Read the model definition and answer for the solid it produces. Units are mm, in the model's axes. A direction names the side the tool comes from. Round coordinates to 2 decimals unless told otherwise and drop trailing zeros. Write each loop counter-clockwise with the first axis right and the second up, starting at its lowest first coordinate (ties: lowest second). Pieces come first, ordered by that corner, then holes. Notation, with made-up numbers: (44.5, 16) -> (99.5, 16) arc R35 cw to (99.5, 55) -> close; hole circle Ø6 at (-28.75, 35.25). An arc over 180 degrees is marked (long way). Return JSON: item names as keys, results as strings.
from build123d import *

# Parameters (mm, degrees)
SKETCH1_W                = 13
SKETCH1_H                = 42
SKETCH1_R                = 1.75
BOSS_EXTRUDE1_DEPTH      = 4
SKETCH1_3_W              = 2
SKETCH1_3_H              = 42
BOSS_EXTRUDE2_DEPTH      = 30
SKETCH3_R                = 3.1
CUT_EXTRUDE1_DEPTH       = 50
RIB1_REACH               = 54.156
SKETCH4_WALL_W           = 135.380915612
SKETCH4_WALL_H           = 2
CUT_EXTRUDE2_DEPTH       = 2.5
BOSS_EXTRUDE3_DEPTH      = 2
BOSS_EXTRUDE3_DEPTH_BACK = 2
SKETCH7_W                = 42
SKETCH7_H                = 30
SKETCH8_R                = 3.05
CUT_EXTRUDE3_DEPTH       = 12


with BuildPart() as part:
    # Sketch1 → Boss-Extrude1 (new body)
    with BuildSketch(Plane(origin=(0, 0, 0), x_dir=(1, 0, 0), z_dir=(0, 1, 0))):
        with Locations((-1, 0)):
            Rectangle(SKETCH1_W, SKETCH1_H)
        with Locations(Location((0.72, -14, 0), (0, 0, 270))):
            Circle(SKETCH1_R, mode=Mode.SUBTRACT)
        with Locations(Location((0.72, 14, 0), (0, 0, 270))):
            Circle(SKETCH1_R, mode=Mode.SUBTRACT)
    extrude(amount=BOSS_EXTRUDE1_DEPTH)

    # Sketch1_3 → Boss-Extrude2 (add)
    with BuildSketch(Plane(origin=(0, 0, 0), x_dir=(1, 0, 0), z_dir=(0, 1, 0))):
        with Locations((6.5, 0)):
            Rectangle(SKETCH1_3_W, SKETCH1_3_H)
    extrude(amount=BOSS_EXTRUDE2_DEPTH)

    # Sketch3 → Cut-Extrude1 (cut)
    with BuildSketch(Plane(origin=(7.5, 0, 0), x_dir=(0, 0, -1), z_dir=(1, 0, 0))):
        with Locations((0, 22.5)):
            Circle(SKETCH3_R)
    extrude(amount=-CUT_EXTRUDE1_DEPTH, mode=Mode.SUBTRACT)

    # Sketch4 wall → Rib1 (add, up to next)
    with BuildSketch(Plane(origin=(-1, 17, 21), x_dir=(0.4472135955, 0.894427191, 0), z_dir=(-0.894427191, 0.4472135955, 0)), mode=Mode.PRIVATE) as rib1_sk1:
        with Locations((0, 1)):
            Rectangle(SKETCH4_WALL_W, SKETCH4_WALL_H)
    rib1_tool1 = extrude(rib1_sk1.sketch, amount=-RIB1_REACH, mode=Mode.PRIVATE) - part.part
    rib1 = rib1_tool1.solids().sort_by_distance((-1, 17, 21))[0]
    add(rib1)

    # Mirror1: Rib1 across plane
    add(rib1.mirror(Plane.XY))

    # Sketch6 → Cut-Extrude2 (cut)
    with BuildSketch(Plane(origin=(0, 4, 0), x_dir=(1, 0, 0), z_dir=(0, 1, 0))):
        Polygon((-2.570896534, -14), (-0.925448267, -16.85), (2.365448267, -16.85), (4.010896534, -14), (2.365448267, -11.15), (-0.925448267, -11.15), align=None)
        Polygon((-2.570896534, 14), (-0.925448267, 11.15), (2.365448267, 11.15), (4.010896534, 14), (2.365448267, 16.85), (-0.925448267, 16.85), align=None)
    extrude(amount=-CUT_EXTRUDE2_DEPTH, mode=Mode.SUBTRACT)

    # Sketch7 → Boss-Extrude3 (add, two sides: drawn at the far end of the back side and taken through both)
    with BuildSketch(Plane(origin=(7.5, 0, 0), x_dir=(0, 0, -1), z_dir=(1, 0, 0)).offset(-BOSS_EXTRUDE3_DEPTH_BACK)):
        with Locations((0, 15)):
            Rectangle(SKETCH7_W, SKETCH7_H)
    extrude(amount=BOSS_EXTRUDE3_DEPTH + BOSS_EXTRUDE3_DEPTH_BACK)

    # Sketch8 → Cut-Extrude3 (cut)
    with BuildSketch(Plane(origin=(9.5, 0, 0), x_dir=(0, 0, -1), z_dir=(1, 0, 0))):
        with Locations((0.5, 22.5)):
            Circle(SKETCH8_R)
    extrude(amount=-CUT_EXTRUDE3_DEPTH, mode=Mode.SUBTRACT)


solid = part.part
Item 1: Section C-C (y = 2.5) is taken. Give the vertices of the cut face in (x, z), then the cut area to 3 significant figures.
Worked answers:
{"outline": "(-7.5, -21) -> (9.5, -21) -> (9.5, 21) -> (-7.5, 21) -> close; hole (-2.57, -14) -> (-0.93, -16.85) -> (2.37, -16.85) -> (4.01, -14) -> (2.37, -11.15) -> (-0.93, -11.15) -> close; hole (-2.57, 14) -> (-0.93, 11.15) -> (2.37, 11.15) -> (4.01, 14) -> (2.37, 16.85) -> (-0.93, 16.85) -> close", "area": "658 mm2"}
Item 2: Section D-D (z = -4.5) is taken. Give the vertices of the cut face in (x, y), then the cut area to 3 significant figures.
Worked answers:
{"outline": "(-7.5, 0) -> (9.5, 0) -> (9.5, 30) -> (5.5, 30) -> (5.5, 4) -> (-7.5, 4) -> close", "area": "172 mm2"}
Item 3: Section A-A (y = 22.5) is taken. Give the vertices of the cut face in (x, z).
Worked answers:
{"outline": "(1.75, -21) -> (9.5, -21) -> (9.5, -3.55) -> (5.5, -3.55) -> (5.5, -19) -> (1.75, -19) -> close; (1.75, 19) -> (5.5, 19) -> (5.5, 2.55) -> (9.5, 2.55) -> (9.5, 21) -> (1.75, 21) -> close"}
Item 4: For a pull along X with two mould halves and no side action, classify faces 4 (the flat face through (-1, 17, -20)), 5 (the cylindrical face through (1.246, 0.74, 15.669)), 6 (the cylindrical face through (7.528, 20.644, 1.92)) as released by +X, released by -X, zero draft, split by the parting line, or undercut.
Worked answers:
{"face 4": "released by -X", "face 5": "undercut", "face 6": "zero draft"}
Item 5: A tool of negligible diameter and unlimited length cuts with its end or side. For faces 1 (the flat face through (-1.76, 2.768, 15.405)), 2 (the flat face through (-1, 17, 20)), 3 (the flat face through (0, 13, -19)), from which of +Z, -Z, +X, -X, +Y, -Y can it reach the whole face along a straight path? Write none if from no direction.
Worked answers:
{"face 1": "+Y", "face 2": "+Z, -Z, -X, +Y", "face 3": "-X, +Y"}
Item 6: Straight lines are drawn through the part: L1, parallel to Z at x = 0.72, y = 0.9; L2, parallel to Z at x = -4, y = 9.75; L3, parallel to Y at x = 7.3, z = -0.5. For each, find the intervals that lie inside material, in ascending order. Write a range as [from, to].
Worked answers:
{"L1": "z = [-21, -15.75], [-12.25, 12.25], [15.75, 21]", "L2": "z = [-21, -19], [19, 21]", "L3": "y = [0, 19.45], [25.55, 30]"}
Item 7: Flat-ended cylindrical pins translate along their axes: pin 1 (4 mm diameter, centred on x = 0.72, z = 14, fed in from +Y); pin 2 (8 mm diameter, centred on x = -3.5, z = -4, fed in from +Y); pin 3 (8 mm diameter, centred on y = 22.5, z = -0.5, fed in from -X). Find the tip coordinate at first contact, or state that the pin passes through.
Worked answers:
{"pin 1": "stops at y = 1.5", "pin 2": "stops at y = 4", "pin 3": "stops at x = 5.5"}
Item 8: Section B-B (x = 0.72) is taken. Give the vertices of the cut face in (y, z), then the cut area to 3 significant figures.
Worked answers:
{"outline": "(0, -21) -> (20.44, -21) -> (20.44, -19) -> (4, -19) -> (4, -16.85) -> (1.5, -16.85) -> (1.5, -15.75) -> (0, -15.75) -> close; (0, -12.25) -> (1.5, -12.25) -> (1.5, -11.15) -> (4, -11.15) -> (4, 11.15) -> (1.5, 11.15) -> (1.5, 12.25) -> (0, 12.25) -> close; (0, 15.75) -> (1.5, 15.75) -> (1.5, 16.85) -> (4, 16.85) -> (4, 19) -> (20.44, 19) -> (20.44, 21) -> (0, 21) -> close", "area": "195 mm2"}
